The listing builds one solid part. Answer for the finished solid, in the listing's coordinates (mm). Round coordinates to 2 decimals unless told otherwise and drop trailing zeros. Loops run counter-clockwise (first coordinate to the right, second up) from the corner with the lowest first, then second, coordinate; pieces in that order, holes last. Notation, with made-up numbers: (-5, 41) -> (3, 41) arc R34 ccw to (3, 74) -> close; hole circle Ø3 at (6, -32). An arc over 180 degrees is marked (long way). Use a Markdown table: item, result. Add a question column.
Q1. Consider line 1 (Y direction, x = -247.65, z = 1.6); line 2 (Y direction, x = -254, z = 0.9); line 3 (X direction, y = 799.5, z = 1.2). Determine where each line is inside the solid, lowest interval first.
Q2. Section C-C on x = -148.5 is taken. Give the vertices of the cut face in (y, z) (3 decimals).
Q3. Section B-B on y = 83.5 is taken. Give the vertices of the cut face in (x, z) (3 decimals).
Q4. Section A-A on z = 1 is taken. Give the vertices of the cut face in (x, y) (3 decimals), then the cut area to 3 significant figures.
Q5. For a pull along Y with two mould halves and no side action, classify faces 1 (the cylindrical face through (-248.72, 728.91, 1.61)), 2 (the flat face through (-199.606, 800.386, 1.565)), 3 (the cylindrical face through (-126.02, 132.92, 1.61)) as released by +Y, released by -Y, zero draft, split by the parting line, or undercut.
from build123d import *

# Parameters (mm, degrees)
BOSS_EXTRUDE1_DEPTH = 3.175
SKETCH5_R           = 8.255
CUT_EXTRUDE3_DEPTH  = 4.175
CUT_EXTRUDE4_DEPTH  = 4.175


with BuildPart() as part:
    # Sketch1 → Boss-Extrude1 (new body)
    with BuildSketch(Plane.XY):
        Polygon((0, 0), (-393.7, 0), (-393.7, 596.9), (0, 1009.65), align=None)
    extrude(amount=BOSS_EXTRUDE1_DEPTH)

    # Sketch5 → Cut-Extrude3 (cut, through all)
    with BuildSketch(Plane.XY.offset(3.175)):
        with Locations((-247.65, 720.725)):
            Circle(SKETCH5_R)
    extrude(amount=-CUT_EXTRUDE3_DEPTH, mode=Mode.SUBTRACT)

    # Sketch6 → Cut-Extrude4 (cut, through all)
    with BuildSketch(Plane.XY.offset(3.175)):
        with BuildLine():
            Line((0, 142.875), (-101.6, 142.875))
            ThreePointArc((-101.6, 142.875), (-126.295704333, 132.645704333), (-136.525, 107.95))
            Line((-136.525, 107.95), (-136.525, 0))
            Line((-136.525, 0), (0, 0))
            Line((0, 0), (0, 142.875))
        make_face()
    extrude(amount=-CUT_EXTRUDE4_DEPTH, mode=Mode.SUBTRACT)


solid = part.part
Checked values:
| question | item | result |
|---|---|---|
| 1 | line 1 | y = 0 to 712.47, 728.98 to 750.02 |
| 1 | line 2 | y = 0 to 715.45, 726 to 743.36 |
| 1 | line 3 | x = -200.45 to 0 |
| 2 | outline | (0, 0) -> (853.965, 0) -> (853.965, 3.175) -> (0, 3.175) -> close |
| 3 | outline | (-393.7, 0) -> (-136.525, 0) -> (-136.525, 3.175) -> (-393.7, 3.175) -> close |
| 4 | outline | (-393.7, 0) -> (-136.525, 0) -> (-136.525, 107.95) arc R34.925 cw to (-101.6, 142.875) -> (0, 142.875) -> (0, 1009.65) -> (-393.7, 596.9) -> close; hole circle Ø16.51 at (-247.65, 720.725) |
| 4 | area | 297,000 mm2 |
| 5 | face 1 | undercut |
| 5 | face 2 | released by +Y |
| 5 | face 3 | released by -Y |
